from build123d import *

# Parameters (mm, degrees)
SKETCH5_W           = 145
SKETCH5_H           = 77
BOSS_EXTRUDE2_DEPTH = 17
CHAMFER2_SIZE       = 63
CHAMFER2_SIZE2      = 10
SKETCH1_R           = 2.6
SKETCH1_R_2         = 1.65
CUT_EXTRUDE1_DEPTH  = 5


with BuildPart() as part:
    # Sketch5 → Boss-Extrude2 (new body)
    with BuildSketch(Plane(origin=(0, 0, 0), x_dir=(1, 0, 0), z_dir=(0, 1, 0))):
        with Locations((72.5, 38.5)):
            Rectangle(SKETCH5_W, SKETCH5_H)
    extrude(amount=BOSS_EXTRUDE2_DEPTH)

    # Chamfer2
    chamfer2_edges = [part.edges().sort_by_distance(p)[0] for p in [
        (72.5, 0, 0),
    ]]
    chamfer2_side = [part.faces().sort_by_distance(p)[0] for p in [
        (72.5, 0, -38.5),
    ]]
    chamfer(chamfer2_edges, length=CHAMFER2_SIZE, length2=CHAMFER2_SIZE2, reference=chamfer2_side[0])

    # Sketch1 → Cut-Extrude1 (cut)
    with BuildSketch(Plane(origin=(0, 17, 0), x_dir=(1, 0, 0), z_dir=(0, 1, 0))):
        with Locations(Location((5, 72, 0), (0, 0, 270))):
            Circle(SKETCH1_R)
        with Locations(Location((5, 5, 0), (0, 0, 270))):
            Circle(SKETCH1_R)
        with Locations(Location((140, 5, 0), (0, 0, 270))):
            Circle(SKETCH1_R)
        with Locations(Location((140, 72, 0), (0, 0, 270))):
            Circle(SKETCH1_R)
        with Locations(Location((46.91, 70, 0), (0, 0, 270))):
            Circle(SKETCH1_R_2)
        with Locations(Location((46.91, 54.76, 0), (0, 0, 270))):
            Circle(SKETCH1_R_2)
        with Locations(Location((98.09, 70, 0), (0, 0, 270))):
            Circle(SKETCH1_R_2)
        with Locations(Location((98.09, 54.76, 0), (0, 0, 270))):
            Circle(SKETCH1_R_2)
    extrude(amount=-CUT_EXTRUDE1_DEPTH, mode=Mode.SUBTRACT)


solid = part.part
The model under review builds one solid part; all positions refer to its coordinate system, in mm. A direction names the side the tool comes from. Round coordinates to 2 decimals unless told otherwise and drop trailing zeros. Write each loop counter-clockwise with the first axis right and the second up, starting at its lowest first coordinate (ties: lowest second). Pieces come first, ordered by that corner, then holes. Notation, with made-up numbers: M -26.5,39 L 32.5,39 A33 cw 32.5,69 Z; hole C 21,44.5 d8. An arc over 180 degrees is marked long. Use a Markdown table: item, result. Add a question column.
Q1. We need section D-D, the plane x = 46.91. State the section outline as (y, z) points.
Q2. We need section A-A, the plane x = 5. State the section outline as (y, z) points, plus the area to 3 significant figures.
Q3. We need section C-C, the plane y = 7.5. State the section outline as (x, z) points.
Q4. Machinability: for faces 5 (the face through (71, 17, -39)), 6 (the face through (46.278, 14.535, -53.236)), which of the approach directions +Z, -Z, +X, -X, +Y, -Y give a long, thin tool a straight path to every point of the face, cutting with its end or side? Answer none if there is none.
Q5. The part is to be moulded in two halves that separate along Z. For faces 1 (the face through (71, 8, -77)), 2 (the face through (145, 10, -47)), 3 (the face through (138.418, 14.535, -74.063)), 4 (the face through (71, 13, 0)), say which applies: pulls with the +Z half, pulls with the -Z half, needs draft (parallel to the pull), parting line crosses it, or undercut.
Q6. We need section B-B, the plane z = -54.76. State the section outline as (x, y) points.
Q7. Insertion check: pin 1 (1.6 mm diameter, centred on x = 5, z = -6, fed in from +Y); pin 2 (6 mm diameter, centred on y = 2.5, z = -9.5, fed in from +X); pin 3 (3 mm diameter, centred on x = 5, z = -5, fed in from -Y). Each pin has a flat end and moves straight along its axis. Give the tip position at first contact, or say it passes through.
Q8. To check wall thickness, follow line 1 (X direction, y = 14.9, z = -5); line 2 (X direction, y = 12.5, z = -3.5); line 3 (Z direction, x = 98.09, y = 15.3). State the ranges of each line that lie inside material, in increasing order.
Findings below:
| question | item | result |
|---|---|---|
| 1 | outline | M 0,-77 L 17,-77 L 17,-71.65 L 12,-71.65 L 12,-68.35 L 17,-68.35 L 17,-56.41 L 12,-56.41 L 12,-53.11 L 17,-53.11 L 17,0 L 10,0 L 0,-63 Z |
| 2 | outline | M 0,-77 L 17,-77 L 17,-74.6 L 12,-74.6 L 12,-69.4 L 17,-69.4 L 17,-7.6 L 12,-7.6 L 12,-2.4 L 17,-2.4 L 17,0 L 10,0 L 0,-63 Z |
| 2 | area | 942 mm² |
| 3 | outline | M 0,-77 L 145,-77 L 145,-15.75 L 0,-15.75 Z |
| 4 | face 5 | +Z, -Z, +X, -X, +Y |
| 4 | face 6 | +Y |
| 5 | face 1 | pulls with the -Z half |
| 5 | face 2 | needs draft |
| 5 | face 3 | undercut |
| 5 | face 4 | pulls with the +Z half |
| 6 | outline | M 0,1.31 L 145,1.31 L 145,17 L 99.74,17 L 99.74,12 L 96.44,12 L 96.44,17 L 48.56,17 L 48.56,12 L 45.26,12 L 45.26,17 L 0,17 Z |
| 7 | pin 1 | stops at y = 12 |
| 7 | pin 2 | passes through |
| 7 | pin 3 | stops at y = 8.97 |
| 8 | line 1 | x = 0 to 2.4, 7.6 to 137.4, 142.6 to 145 |
| 8 | line 2 | x = 0 to 2.88, 7.12 to 137.88, 142.12 to 145 |
| 8 | line 3 | z = -77 to -71.65, -68.35 to -56.41, -53.11 to 0 |
